Study the drawing (mm; zero at the part's minimum x, y, z) and answer. A direction names the side the tool comes from. Coordinates: 2 decimals unless noted, no trailing zeros. Order: outer loops, then holes, each group sorted by start corner. A loop starts at its lowest first (then second) coordinate and runs counter-clockwise, first axis right, second up. Notation, with made-up numbers: (-27, -15) -> (6, -15) arc R34 cw to (6, 20) -> close; hole circle Ø11 at (-16, -27). An arc over 180 degrees is marked (long way). One line per question, with ' | ' between items.
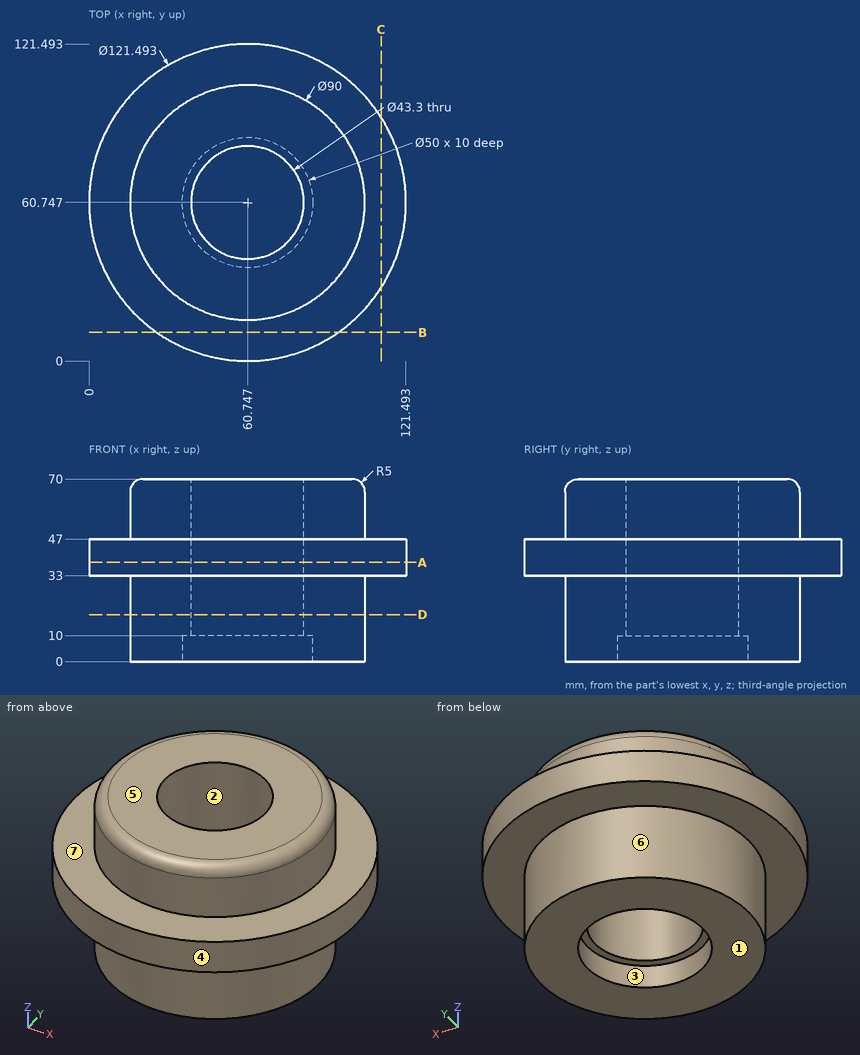
Item 1: Determine the mould class of the marked faces 1, 2, 3 and 4 for opening direction Y: pulls with the +Y half, pulls with the -Y half, needs draft (parallel to the pull), parting line crosses it, or undercut.
Computed values:
face 1: needs draft | face 2: undercut | face 3: undercut | face 4: parting line crosses it
Item 2: Section C-C, the plane x = 112 is taken. Give the vertices of the cut face in (y, z) (1 decimal).
Computed values:
outline: (28.1, 33) -> (93.4, 33) -> (93.4, 47) -> (28.1, 47) -> close
Item 3: For the marked faces 5, 6 and 7, determine the directions among +Z, -Z, +X, -X, +Y, -Y from which every point of the face is accessible in a straight line to the end or side of a thin tool.
Computed values:
face 5: +Z, +X, -X, +Y, -Y | face 6: -Z | face 7: +Z
Item 4: Section B-B, the plane y = 11 is taken. Give the vertices of the cut face in (x, z).
Computed values:
outline: (25.88, 33) -> (95.61, 33) -> (95.61, 47) -> (25.88, 47) -> close
Item 5: Section D-D, the plane z = 18 is taken. Give the vertices of the cut face in (x, y), plus the area to 3 significant figures.
Computed values:
outline: circle Ø90 at (60.75, 60.75); hole circle Ø43.3 at (60.75, 60.75) | area: 4,890 mm^2
Item 6: Each of these flat-tipped pins is pushed along its axis until it touches: pin 1 Ø5 at (x, z) = (21.5, 32.5) entering from -Y; pin 2 Ø3 at (x, y) = (94, 101) entering from +Z; pin 3 Ø1.5 at (x, z) = (91.5, 36) entering from -Y; pin 4 Ø8 at (x, y) = (57.5, 105.5) entering from -Z. Where does it stop, or does it pass through?
Computed values:
pin 1: stops at y = 12.41 | pin 2: stops at z = 47 | pin 3: stops at y = 7.93 | pin 4: stops at z = 0
Item 7: Section A-A, the plane z = 38 is taken. Give the vertices of the cut face in (x, y).
Computed values:
outline: circle Ø121.49 at (60.75, 60.75); hole circle Ø43.3 at (60.75, 60.75)
Item 8: Find the intervals of material crossed by L1, parallel to Z at x = 100, y = 83; L2, parallel to X at y = 53.5, z = 16.5 (1 decimal); L3, parallel to Y at x = 68.5, z = 9.5 (1 decimal), in increasing order.
Computed values:
L1: z = 33 to 47 | L2: x = 16.3 to 40.3, 81.1 to 105.2 | L3: y = 16.4 to 37, 84.5 to 105.1
